Source: three-view drawing plus pictorial views. Frame: mm from the lowest corner of the part. Give positions to 0.01 mm unless a question says otherwise; leave off trailing zeros. Order: outer loops, then holes, each group sorted by start corner. A loop starts at its lowest first (then second) coordinate and runs counter-clockwise, first axis right, second up. Notation, with made-up numbers: M 71,83 L 93,83 A26 ccw 93,121 Z; hole C -23,58.25 d11. An arc over 180 degrees is marked long. Use CSV: the item, a comma, the result in double quotes. Start each with the question number.
1. Pin query (flat end, axial travel): P1, Ø2, axis at x = 3.5, z = 4, coming from the +Y side. Return the tip coordinate at first contact, or that it passes through.
2. Section query C-C, the plane y = 0.25. Return the cut outline in (x, z).
3. Section query A-A, the plane x = 3.75. Return the cut outline in (y, z).
4. Line query: line 1 along X through (y, z) = (0.3, 4); line 2 along Z through (x, y) = (11.25, 0.55); line 3 along X through (y, z) = (0.7, 4.25). Output: solid intervals per line, ascending. Write a range as [from, to].
5. Section query B-B, the plane z = 4. Return the cut outline in (x, y), plus the area to 3 significant figures.
6. Mould query, pull axis X, two halves, no side actions, for the marked faces 1, 2 and 3. Classes: released by +X, released by -X, zero draft, split by the parting line, or undercut.
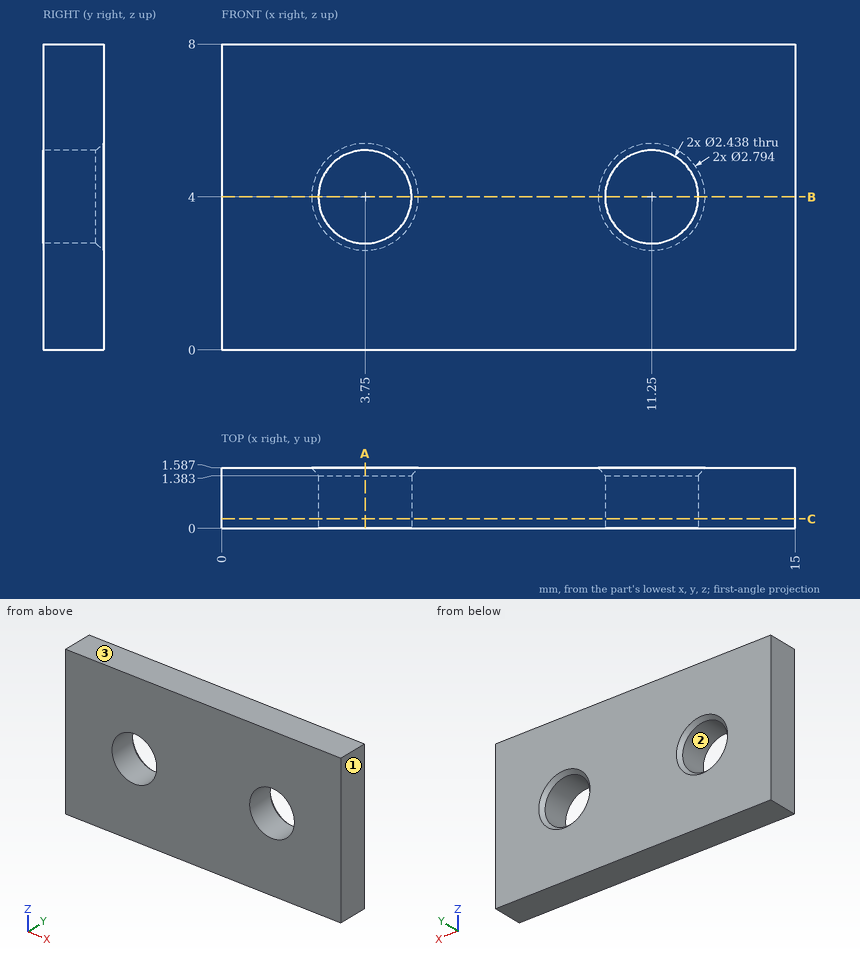
Result set:
1,P1,"y = 1.42"
2,outline,"M 0,0 L 15,0 L 15,8 L 0,8 Z; hole C 3.75,4 d2.44; hole C 11.25,4 d2.44"
3,outline,"M 0,0 L 1.59,0 L 1.59,2.6 L 1.38,2.78 L 0,2.78 Z; M 0,5.22 L 1.38,5.22 L 1.59,5.4 L 1.59,8 L 0,8 Z"
4,line 1,"[0, 2.53], [4.97, 10.03], [12.47, 15]"
4,line 2,"[0, 2.78], [5.22, 8]"
4,line 3,"[0, 2.56], [4.94, 10.06], [12.44, 15]"
5,outline,"M 0,0 L 2.53,0 L 2.53,1.38 L 2.35,1.59 L 0,1.59 Z; M 4.97,0 L 10.03,0 L 10.03,1.38 L 9.85,1.59 L 5.15,1.59 L 4.97,1.38 Z; M 12.47,0 L 15,0 L 15,1.59 L 12.65,1.59 L 12.47,1.38 Z"
5,area,"16.0 mm2"
6,face 1,"released by +X"
6,face 2,"undercut"
6,face 3,"zero draft"
